For this review, take the finished solid that the model builds, in its own axes (mm). Face numbers are marked on the shaded views. A direction names the side the tool comes from. Coordinates: 2 decimals unless noted, no trailing zeros. Order: outer loops, then holes, each group sorted by start corner. A loop starts at its lowest first (then second) coordinate and runs counter-clockwise, first axis right, second up. Notation, with made-up numbers: (57, -14) -> (82, -14) arc R19 ccw to (82, 3) -> close; hole circle Ø3 at (63, 60.5). An arc over 180 degrees is marked (long way). Answer as a JSON object with one key per item and string values. Group by question number.
1) Add section C-C, the plane y = 9. Count the separate pieces of the cut face and the enclosed holes in it, then the cut area to 3 significant figures.
2) Add section A-A, the plane z = -77. Write out the cut boundary in (x, y), then the cut area to 3 significant figures.
3) Add section B-B, the plane x = 72. Write out the cut boundary in (y, z).
4) For pin 1 (3 mm diameter, centred on x = 59, y = 2, fed in from +Z); pin 2 (10 mm diameter, centred on x = 56, z = -44, fed in from -Y); pin 3 (1 mm diameter, centred on x = 53, z = 1.5, fed in from -Y), all flat-tipped, find the tip position at first contact; note any pin that passes through.
5) Wall thickness on L1, parallel to X at y = 8.25, z = 10; L2, parallel to X at y = 17.1, z = -77; L3, parallel to Z at x = 36, y = 10.5: over which ranges is each line inside the solid? List them lowest first.
6) Machinability: for the marked faces 4 and 5, which of the approach directions +Z, -Z, +X, -X, +Y, -Y give a long, thin tool a straight path to every point of the face, cutting with its end or side? Answer none if there is none.
7) Add section D-D, the plane z = -58.5. Write out the cut boundary in (x, y), then the cut area to 3 significant figures.
8) Draft analysis for pull direction X (two halves, no side actions). For the marked faces 1, 2 and 3, state which applies: +X half, -X half, draft (parallel to the pull), parting line (faces both ways), or undercut.
from build123d import *

# Parameters (mm, degrees)
SKETCH_1_R          = 2.1
EXTRUDE_1_DEPTH     = 16
SKETCH_2_R          = 2.1
EXTRUDE_2_DEPTH     = 2
EXTRUDE_START       = -2
EXTRUDE_3_DEPTH     = 2
SKETCH_4_W          = 5.8
SKETCH_4_H          = 13.4
CUT_EXTRUDE_1_DEPTH = 2
SKETCH_5_W          = 9
SKETCH_5_H          = 11
CUT_EXTRUDE_2_DEPTH = 2
SKETCH_6_W          = 16.7
SKETCH_6_H          = 18
CUT_EXTRUDE_3_DEPTH = 15.5
SKETCH_7_R          = 1.6
CUT_EXTRUDE_4_DEPTH = 2


with BuildPart() as part:
    # 草图1 → 凸台-拉伸1 (new body)
    with BuildSketch(Plane(origin=(0, 0, 0), x_dir=(1, 0, 0), z_dir=(0, 1, 0))):
        with BuildLine():
            Line((41.776260997, -10), (41.776260997, -2.5))
            Line((41.776260997, -2.5), (151.776260997, -2.5))
            Line((151.776260997, -2.5), (151.776260997, -10))
            ThreePointArc((151.776260997, -10), (153.53362031, -14.242640687), (157.776260997, -16))
            ThreePointArc((157.776260997, -16), (162.018901684, -14.242640687), (163.776260997, -10))
            Line((163.776260997, -10), (163.776260997, 90))
            ThreePointArc((163.776260997, 90), (162.018901684, 94.242640687), (157.776260997, 96))
            Line((157.776260997, 96), (35.776260997, 96))
            ThreePointArc((35.776260997, 96), (31.53362031, 94.242640687), (29.776260997, 90))
            Line((29.776260997, 90), (29.776260997, -10))
            ThreePointArc((29.776260997, -10), (31.53362031, -14.242640687), (35.776260997, -16))
            ThreePointArc((35.776260997, -16), (40.018901684, -14.242640687), (41.776260997, -10))
        make_face()
        with Locations(Location((35.776260997, -10, 0), (0, 0, 270))):
            Circle(SKETCH_1_R, mode=Mode.SUBTRACT)
        with Locations(Location((35.776260997, 90, 0), (0, 0, 270))):
            Circle(SKETCH_1_R, mode=Mode.SUBTRACT)
        with Locations(Location((157.776260997, 90, 0), (0, 0, 270))):
            Circle(SKETCH_1_R, mode=Mode.SUBTRACT)
        with Locations(Location((157.776260997, -10, 0), (0, 0, 270))):
            Circle(SKETCH_1_R, mode=Mode.SUBTRACT)
        with BuildLine():
            Line((31.776260997, -0.5), (161.776260997, -0.5))
            Line((161.776260997, -0.5), (161.776260997, 80.5))
            Line((161.776260997, 80.5), (157.776260997, 80.5))
            Line((157.776260997, 80.5), (157.776260997, 84))
            ThreePointArc((157.776260997, 84), (152.299035422, 87.550510257), (153.304125042, 94))
            Line((153.304125042, 94), (96.776260997, 94))
            Line((96.776260997, 94), (40.248396952, 94))
            ThreePointArc((40.248396952, 94), (41.253486572, 87.550510257), (35.776260997, 84))
            Line((35.776260997, 84), (35.776260997, 80.5))
            Line((35.776260997, 80.5), (31.776260997, 80.5))
            Line((31.776260997, 80.5), (31.776260997, -0.5))
        make_face(mode=Mode.SUBTRACT)
    extrude(amount=EXTRUDE_1_DEPTH)

    # 草图2 → 凸台-拉伸2 (add)
    with BuildSketch(Plane(origin=(0, 16, 0), x_dir=(1, 0, 0), z_dir=(0, 1, 0))):
        with BuildLine():
            Line((29.776260997, 90), (29.776260997, -10))
            ThreePointArc((29.776260997, -10), (35.776260997, -16), (41.776260997, -10))
            Line((41.776260997, -10), (41.776260997, -2.5))
            Line((41.776260997, -2.5), (151.776260997, -2.5))
            Line((151.776260997, -2.5), (151.776260997, -10))
            ThreePointArc((151.776260997, -10), (157.776260997, -16), (163.776260997, -10))
            Line((163.776260997, -10), (163.776260997, 90))
            ThreePointArc((163.776260997, 90), (162.018901684, 94.242640687), (157.776260997, 96))
            Line((157.776260997, 96), (35.776260997, 96))
            ThreePointArc((35.776260997, 96), (31.53362031, 94.242640687), (29.776260997, 90))
        make_face()
        with Locations(Location((35.776260997, 90, 0), (0, 0, 270))):
            Circle(SKETCH_2_R, mode=Mode.SUBTRACT)
        with Locations(Location((157.776260997, 90, 0), (0, 0, 270))):
            Circle(SKETCH_2_R, mode=Mode.SUBTRACT)
        with Locations(Location((35.776260997, -10, 0), (0, 0, 270))):
            Circle(SKETCH_2_R, mode=Mode.SUBTRACT)
        with Locations(Location((157.776260997, -10, 0), (0, 0, 270))):
            Circle(SKETCH_2_R, mode=Mode.SUBTRACT)
    extrude(amount=EXTRUDE_2_DEPTH)

    # 草图3 → 凸台-拉伸3 (add)
    with BuildSketch(Plane(origin=(0, 18, 0), x_dir=(1, 0, 0), z_dir=(0, 1, 0)).offset(EXTRUDE_START)):
        with BuildLine():
            Line((41.776260997, -2.5), (151.776260997, -2.5))
            Line((151.776260997, -2.5), (151.776260997, -10))
            ThreePointArc((151.776260997, -10), (153.53362031, -14.242640687), (157.776260997, -16))
            Line((157.776260997, -16), (35.776260997, -16))
            ThreePointArc((35.776260997, -16), (40.018901684, -14.242640687), (41.776260997, -10))
            Line((41.776260997, -10), (41.776260997, -2.5))
        make_face()
    extrude(amount=EXTRUDE_3_DEPTH)

    # 草图4 → 切除-拉伸1 (cut)
    with BuildSketch(Plane.XY.offset(2.5)):
        with Locations((67.676260997, 6.7)):
            Rectangle(SKETCH_4_W, SKETCH_4_H)
        with Locations((53.676260997, 6.7)):
            Rectangle(SKETCH_4_W, SKETCH_4_H)
        with Locations((81.676260997, 6.7)):
            Rectangle(SKETCH_4_W, SKETCH_4_H)
        with Locations((95.676260997, 6.7)):
            Rectangle(SKETCH_4_W, SKETCH_4_H)
        with Locations((109.676260997, 6.7)):
            Rectangle(SKETCH_4_W, SKETCH_4_H)
        with Locations((123.676260997, 6.7)):
            Rectangle(SKETCH_4_W, SKETCH_4_H)
        with Locations((137.676260997, 6.7)):
            Rectangle(SKETCH_4_W, SKETCH_4_H)
    extrude(amount=-CUT_EXTRUDE_1_DEPTH, mode=Mode.SUBTRACT)

    # 草图5 → 切除-拉伸2 (cut)
    with BuildSketch(Plane.ZY.offset(-29.776260997)):
        with Locations((-23, 5.5)):
            Rectangle(SKETCH_5_W, SKETCH_5_H)
    extrude(amount=-CUT_EXTRUDE_2_DEPTH, mode=Mode.SUBTRACT)

    # 草图6 → 切除-拉伸3 (cut)
    with BuildSketch(Plane.ZY.offset(-29.776260997)):
        with Locations((-46.65, 9)):
            Rectangle(SKETCH_6_W, SKETCH_6_H)
    extrude(amount=-CUT_EXTRUDE_3_DEPTH, mode=Mode.SUBTRACT)

    # 草图7 → 切除-拉伸4 (cut)
    with BuildSketch(Plane(origin=(0, 18, 0), x_dir=(1, 0, 0), z_dir=(0, 1, 0))):
        with Locations(Location((158.276260997, 77, 0), (0, 0, 270))):
            Circle(SKETCH_7_R)
        with Locations(Location((35.276260997, 77, 0), (0, 0, 270))):
            Circle(SKETCH_7_R)
        with Locations(Location((35.276260997, 3, 0), (0, 0, 270))):
            Circle(SKETCH_7_R)
        with Locations(Location((158.276260997, 3, 0), (0, 0, 270))):
            Circle(SKETCH_7_R)
    extrude(amount=-CUT_EXTRUDE_4_DEPTH, mode=Mode.SUBTRACT)


solid = part.part
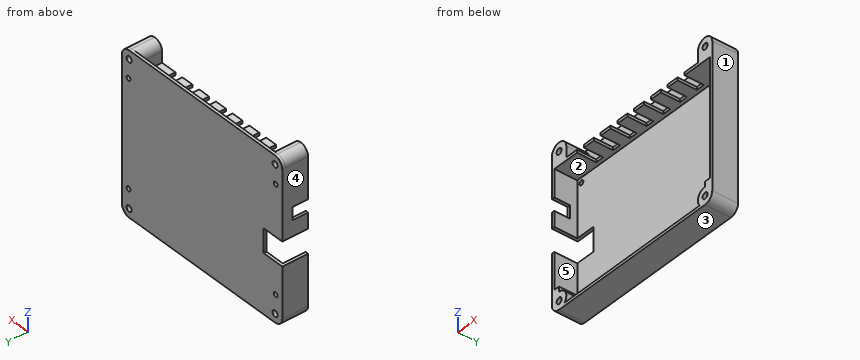
Output values:
{
 "1": {"separate pieces": "9", "enclosed holes": "4", "area": "1,210 mm²"},
 "2": {"outline": "(29.78, 0) -> (31.78, 0) -> (31.78, 16) -> (33.68, 16) -> (33.68, 18) -> (29.78, 18) -> close; (36.88, 16) -> (156.68, 16) -> (156.68, 18) -> (36.88, 18) -> close; (159.88, 16) -> (161.78, 16) -> (161.78, 0) -> (163.78, 0) -> (163.78, 18) -> (159.88, 18) -> close", "area": "319 mm²"},
 "3": {"outline": "(0, -96) -> (18, -96) -> (18, 16) -> (16, 16) -> (16, 2.5) -> (0, 2.5) -> (0, 0.5) -> (16, 0.5) -> (16, -94) -> (0, -94) -> close"},
 "4": {"pin 1": "stops at z = 2.5", "pin 2": "stops at y = 16", "pin 3": "stops at y = 13.4"},
 "5": {"L1": "x = 29.78 to 33.68, 37.88 to 41.78, 151.78 to 155.68, 159.88 to 163.78", "L2": "x = 29.78 to 33.68, 36.88 to 156.68, 159.88 to 163.78", "L3": "z = -96 to -92.09, -87.91 to -84, 0.5 to 7.91, 12.09 to 16"},
 "6": {"face 4": "+Z, -Z, -X, +Y, -Y", "face 5": "-Y"},
 "7": {"outline": "(29.78, 0) -> (31.78, 0) -> (31.78, 16) -> (161.78, 16) -> (161.78, 0) -> (163.78, 0) -> (163.78, 18) -> (29.78, 18) -> close", "area": "332 mm²"},
 "8": {"face 1": "+X half", "face 2": "undercut", "face 3": "draft"}
}
